Geometry: final body of the model. Coordinates: model frame, mm. Round coordinates to 2 decimals unless told otherwise and drop trailing zeros. Write each loop counter-clockwise with the first axis right and the second up, starting at its lowest first coordinate (ties: lowest second). Pieces come first, ordered by that corner, then holes.
from build123d import *

# Parameters (mm, degrees)
SKETCH2_W                    = 82.55
SKETCH2_H                    = 1
F_10_0_1935_DIAMETER_HOLE1_D = 4.9149
CIRPATTERN3_COUNT            = 4
F_10_0_1935_DIAMETER_HOLE2_D = 4.9149


with BuildPart() as part:
    # Sketch2 → Revolve1 (revolve)
    with BuildSketch(Plane(origin=(0, 0, 0), x_dir=(0, 0, -1), z_dir=(1, 0, 0))):
        with Locations((-41.275, 0.5)):
            Rectangle(SKETCH2_W, SKETCH2_H)
    revolve(axis=Axis((0, -0.05, 0), (0, 1, 0)))

    # #10 (0.1935) Diameter Hole1 (through all)
    with Locations(Plane(origin=(0, 1, 0), x_dir=(1, 0, 0), z_dir=(0, 1, 0))):
        with Locations((-25.333643223, 61.160825052), (264.743675233, 73.787758551), (-67.027460084, 27.763683018), (-25.809397513, 25.809397513)):
            f_10_0_1935_diameter_hole1 = Hole(F_10_0_1935_DIAMETER_HOLE1_D / 2)

    # CirPattern3: #10 (0.1935) Diameter Hole1 ×4 about axis
    cirpattern3_axis = Axis((0, 0, 0), (0, 1, 0))
    for i in range(1, CIRPATTERN3_COUNT):
        add(f_10_0_1935_diameter_hole1.rotate(cirpattern3_axis, i * 360 / CIRPATTERN3_COUNT), mode=Mode.SUBTRACT)

    # #10 (0.1935) Diameter Hole2 (through all)
    with Locations(Plane(origin=(0, 1, 0), x_dir=(1, 0, 0), z_dir=(0, 1, 0))):
        with Locations((0, 0)):
            Hole(F_10_0_1935_DIAMETER_HOLE2_D / 2)


solid = part.part
1) Section D-D on z = -52.5. Output: boundary loops of the cut face in (x, y).
2) Draft query along X for faces 1 (the flat face through (-17, 1, -1)), 2 (the cylindrical face through (64.572, 0.493, 27.872)), 3 (the cylindrical face through (-80.587, 0.507, -17.895)). Return one class per face: pulls with the +X half, pulls with the -X half, needs draft (parallel to the pull), parting line crosses it, or undercut.
3) Section B-B on x = 0. Output: boundary loops of the cut face in (y, z), plus the area to 3 significant figures.
4) Section A-A on z = 0. Output: boundary loops of the cut face in (x, y).
5) Line query: probe 1 along X at (y, z) = (0.15, 60.5); probe 2 along X at (y, z) = (0.8, -61.5); probe 3 along Z at (x, y) = (29.5, 0.3). Output: solid intervals per line, ascending.
6) Section C-C on y = 0.75. State how many separate pieces and enclosed holes the cut face has, plus the area to 3 significant figures.
Filled in:
1. outline: (-63.7, 0) - (63.7, 0) - (63.7, 1) - (-63.7, 1) - close
2. face 1: needs draft
2. face 2: undercut
2. face 3: parting line crosses it
3. outline: (0, -82.55) - (1, -82.55) - (1, -2.46) - (0, -2.46) - close; (0, 2.46) - (1, 2.46) - (1, 82.55) - (0, 82.55) - close
3. area: 160 mm2
4. outline: (-82.55, 0) - (-2.46, 0) - (-2.46, 1) - (-82.55, 1) - close; (2.46, 0) - (82.55, 0) - (82.55, 1) - (2.46, 1) - close
5. probe 1: x = -56.16 to 22.97, 27.7 to 56.16
5. probe 2: x = -55.07 to -27.77, -22.9 to 55.07
5. probe 3: z = -77.1 to -68.77, -65.29 to 77.1
6. separate pieces: 1
6. enclosed holes: 13
6. area: 21,200 mm2
